Input: part model. Units: mm. Frame: model coordinates. Face numbers are marked on the shaded views. Give positions to 0.01 mm unless a question says otherwise; leave off trailing zeros. Loops run counter-clockwise (first coordinate to the right, second up) from the corner with the lowest first, then second, coordinate; pieces in that order, holes last. Notation, with made-up numbers: M 32.5,-3 L 83.5,-3 A22 cw 83.5,11 Z; hole C 35.25,12 d1. An arc over 180 degrees is marked long. Answer as a JSON object with one key per item and string values. Group by question number.
1) Ray query, L1, parallel to Y at x = 0, z = 2.35; L2, parallel to Z at x = -7.5, y = 2; L3, parallel to Y at x = 7, z = 1.75. Return the intervals inside material, ascending.
2) Section query C-C on y = -7. Return loops of the section in (x, z), plus the area to 3 significant figures.
3) Section query A-A on x = 0. Return loops of the section in (y, z), plus the area to 3 significant figures.
4) Section query D-D on z = 1.5. Return loops of the section in (x, y).
5) First-contact query: P1, Ø3, axis at x = 4.5, y = -6.5, coming from the -Z side; P2, Ø1.5, axis at x = 9, z = 1.5, coming from the +Y side; P3, Ø1, axis at x = 6.5, z = 0.5, coming from the -Y side. Flat tips, straight axial feed; report the tip coordinate or a pass-through.
6) Draft query along Y for the marked faces 1, 2 and 3. Return one class per face: +Y half, -Y half, draft (parallel to the pull), parting line (faces both ways), or undercut.
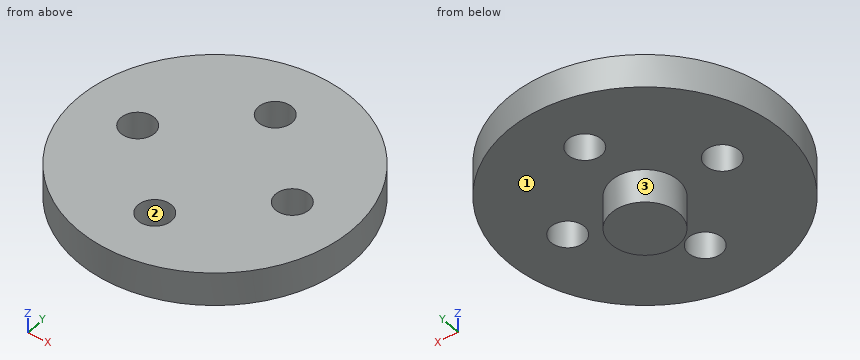
from build123d import *

# Parameters (mm, degrees)
SKETCH2_R           = 12.3
SKETCH2_R_2         = 1.5
BOSS_EXTRUDE1_DEPTH = 3
SKETCH3_R           = 3
BOSS_EXTRUDE2_DEPTH = 3


with BuildPart() as part:
    # Sketch2 → Boss-Extrude1 (new body)
    with BuildSketch(Plane.XY):
        Circle(SKETCH2_R)
        with Locations((-7, 0)):
            Circle(SKETCH2_R_2, mode=Mode.SUBTRACT)
        with Locations((0, 7)):
            Circle(SKETCH2_R_2, mode=Mode.SUBTRACT)
        with Locations((7, 0)):
            Circle(SKETCH2_R_2, mode=Mode.SUBTRACT)
        with Locations((0, -7)):
            Circle(SKETCH2_R_2, mode=Mode.SUBTRACT)
    extrude(amount=BOSS_EXTRUDE1_DEPTH)

    # Sketch3 → Boss-Extrude2 (add)
    with BuildSketch(Plane(origin=(0, 0, 0), x_dir=(-1, 0, 0), z_dir=(0, 0, -1))):
        Circle(SKETCH3_R)
    extrude(amount=BOSS_EXTRUDE2_DEPTH)


solid = part.part
Output:
{
 "1": {"L1": "y = -12.3 to -8.5, -5.5 to 5.5, 8.5 to 12.3", "L2": "z = 0 to 3", "L3": "y = -10.11 to -1.5, 1.5 to 10.11"},
 "2": {"outline": "M -10.11,0 L -1.5,0 L -1.5,3 L -10.11,3 Z; M 1.5,0 L 10.11,0 L 10.11,3 L 1.5,3 Z", "area": "51.7 mm^2"},
 "3": {"outline": "M -12.3,0 L -8.5,0 L -8.5,3 L -12.3,3 Z; M -5.5,0 L -3,0 L -3,-3 L 3,-3 L 3,0 L 5.5,0 L 5.5,3 L -5.5,3 Z; M 8.5,0 L 12.3,0 L 12.3,3 L 8.5,3 Z", "area": "73.8 mm^2"},
 "4": {"outline": "C 0,0 d24.6; hole C -7,0 d3; hole C 0,-7 d3; hole C 0,7 d3; hole C 7,0 d3"},
 "5": {"P1": "stops at z = 0", "P2": "stops at y = 9.12", "P3": "stops at y = -10.74"},
 "6": {"face 1": "draft", "face 2": "undercut", "face 3": "parting line"}
}
